Can you work these out from the model? Positions are in its coordinate system, mm. Face numbers are marked on the shaded views. A direction names the side the tool comes from. Round coordinates to 2 decimals unless told otherwise and drop trailing zeros. Loops run counter-clockwise (first coordinate to the right, second up) from the corner with the lowest first, then second, coordinate; pieces in that order, holes last. Notation, with made-up numbers: M -13,40.25 L 21,40.25 A7 cw 21,51.25 Z; hole C -13,-3 d8. An arc over 180 degrees is marked long. Use a Markdown table: item, result. Add a question column.
```python
from build123d import *

# Parameters (mm, degrees)
F0_W     = 600
F0_H     = 600
F1_DEPTH = 60
F2_W     = 79.0521234274
F2_H     = 79.0521234274
F3_DEPTH = 400
F4_R     = 60
F5_R     = 10


with BuildPart() as f1:
    # F0 (on Top) → F1 (new body)
    with BuildSketch(Plane.XY):
        Rectangle(F0_W, F0_H)
    extrude(amount=F1_DEPTH)

    # F2 (on face) → F3 (join)
    with BuildSketch(Plane(origin=(0, 0, 0), x_dir=(1, 0, 0), z_dir=(0, 0, -1))):
        with Locations((-260.4739382863, 260.4739382863)):
            Rectangle(F2_W, F2_H)
        with Locations((260.4739382863, 260.4739382863)):
            Rectangle(F2_W, F2_H)
        with Locations((-260.4739382863, -260.4739382863)):
            Rectangle(F2_W, F2_H)
        with Locations((260.4739382863, -260.4739382863)):
            Rectangle(F2_W, F2_H)
    extrude(amount=F3_DEPTH)

    # F4
    f4_edges = [f1.edges().sort_by_distance(p)[0] for p in [
        (-300, -300, -170),
        (-300, 300, -170),
        (300, 300, -170),
        (300, -300, -170),
    ]]
    fillet(f4_edges, radius=F4_R)

    # F5
    f5_edges = [f1.edges().sort_by_distance(p)[0] for p in [
        (0, 300, 60),
        (0, 300, 0),
        (220.947877, 300, -200),
        (-220.947877, 300, -200),
        (-300, 0, 0),
        (-300, 220.947877, -200),
        (-300, -220.947877, -200),
        (0, -300, 0),
        (-220.947877, -300, -200),
        (220.947877, -300, -200),
        (300, 0, 0),
        (300, -220.947877, -200),
        (300, 220.947877, -200),
    ]]
    fillet(f5_edges, radius=F5_R)


solid = f1.part
```
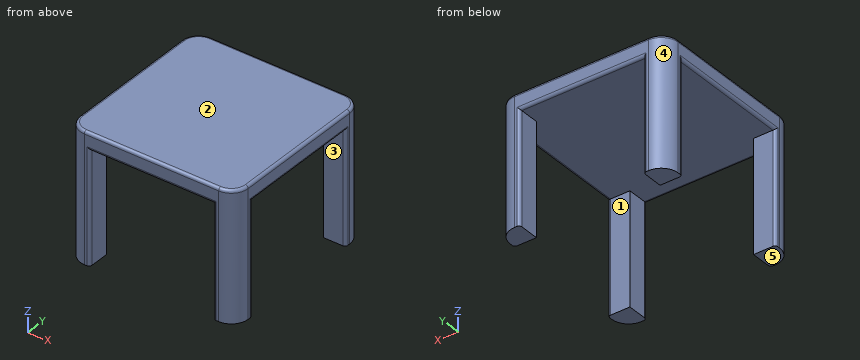
(1) If I drill on probe 1 along Y at (x, z) = (273, -244.5); probe 2 along Z at (x, y) = (246.5, -90); probe 3 along Y at (x, z) = (251, -188), over which ranges is the centre line in solid material (lowest first)? Write a range as [from, to].
(2) On a 3-axis mill with a long thin cutter (end or side, diameter ignored), from which of +Z, -Z, +X, -X, +Y, -Y can I reach the whole of each face in a straight line? I mean the marked faces 1 and 2. Say none if no direction works.
(3) I'm going to push a flat-ended pin straight in: pin 1 (2 mm diameter, centred on x = 183, y = 31.5, fed in from -Z). Where does the tip first touch, or does it pass through?
(4) Suppose I cut it at B-B on x = 165. List the corners of the cut face in (y, z) for me, and give its area (3 significant figures).
(5) Suppose I cut it at A-A on z = -332.5. List the corners of the cut face in (x, y) for me, and give its area (3 significant figures).
(6) Thinking about a two-plate mould opening in Y: for the marked faces 3, 4 and 5, which applies, released by +Y, released by -Y, zero draft, split by the parting line, or undercut?
Results below:
| question | item | result |
|---|---|---|
| 1 | probe 1 | y = [-290.11, -220.95], [220.95, 290.11] |
| 1 | probe 2 | z = [0, 60] |
| 1 | probe 3 | y = [-298.98, -220.95], [220.95, 298.98] |
| 2 | face 1 | -Z, +X, -X |
| 2 | face 2 | +Z, +X, -X, +Y, -Y |
| 3 | pin 1 | stops at z = 0 |
| 4 | outline | M -300,10 A10 ccw -290,0 L 290,0 A10 ccw 300,10 L 300,50 A10 ccw 290,60 L -290,60 A10 ccw -300,50 Z |
| 4 | area | 35,900 mm² |
| 5 | outline | M -300,-240 A60 ccw -240,-300 L -230.95,-300 A10 ccw -220.95,-290 L -220.95,-220.95 L -290,-220.95 A10 ccw -300,-230.95 Z; M -300,230.95 A10 ccw -290,220.95 L -220.95,220.95 L -220.95,290 A10 ccw -230.95,300 L -240,300 A60 ccw -300,240 Z; M 220.95,-290 A10 ccw 230.95,-300 L 240,-300 A60 ccw 300,-240 L 300,-230.95 A10 ccw 290,-220.95 L 220.95,-220.95 Z; M 220.95,220.95 L 290,220.95 A10 ccw 300,230.95 L 300,240 A60 ccw 240,300 L 230.95,300 A10 ccw 220.95,290 Z |
| 5 | area | 21,700 mm² |
| 6 | face 3 | undercut |
| 6 | face 4 | released by +Y |
| 6 | face 5 | zero draft |
